from build123d import *

# Parameters (mm, degrees)
F0_W     = 82.55
F0_H     = 190.5
F1_DEPTH = 19.05
F2_W     = 82.55
F2_H     = 25.4
F3_DEPTH = 73.025
F4_R     = 41.27499
F5_R     = 17.4625
F6_DEPTH = 25.4
F8_DEPTH = 25.4


# Not quite as in the source:
# - a fillet or chamfer is up to 0.001 mm smaller than in the source, because OpenCascade refuses the exact size


with BuildPart() as f1:
    # F0 (on Top) → F1 (new body)
    with BuildSketch(Plane.XY):
        with Locations((41.275, 95.25)):
            Rectangle(F0_W, F0_H)
    extrude(amount=F1_DEPTH)

    # F2 (on face) → F3 (join)
    with BuildSketch(Plane.XY.offset(19.05)):
        with Locations((41.275, 177.8)):
            Rectangle(F2_W, F2_H)
    extrude(amount=F3_DEPTH)

    # F4 (radius 41.275 in the source; OpenCascade refuses exactly that, so slightly less here)
    f4_edges = [f1.edges().sort_by_distance(p)[0] for p in [
        (0, 177.8, 92.075),
        (82.55, 177.8, 92.075),
    ]]
    fillet(f4_edges, radius=F4_R)

    # F5 (on face) → F6 (cut)
    with BuildSketch(Plane.XZ.offset(-165.1)):
        with Locations((41.275, 50.8)):
            Circle(F5_R)
    extrude(amount=-F6_DEPTH, mode=Mode.SUBTRACT)

    # F7 (on face) → F8 (cut)
    with BuildSketch(Plane.XY.offset(19.05)):
        with BuildLine():
            ThreePointArc((58.7375, 114.3), (28.9271478335, 126.6478521665), (41.275, 96.8375))
            ThreePointArc((41.275, 96.8375), (53.6228521665, 101.9521478335), (58.7375, 114.3))
        make_face()
        with BuildLine():
            Line((41.275, 38.1), (41.275, 20.6375))
            ThreePointArc((41.275, 20.6375), (53.6228521665, 25.7521478335), (58.7375, 38.1))
            ThreePointArc((58.7375, 38.1), (53.6228521665, 50.4478521665), (41.275, 55.5625))
            Line((41.275, 55.5625), (41.275, 38.1))
        make_face()
        with BuildLine():
            ThreePointArc((41.275, 55.5625), (23.8125, 38.1), (41.275, 20.6375))
            Line((41.275, 20.6375), (41.275, 38.1))
            Line((41.275, 38.1), (41.275, 55.5625))
        make_face()
    extrude(amount=-F8_DEPTH, mode=Mode.SUBTRACT)


solid = f1.part
The model under review builds one solid part; all positions refer to its coordinate system, in mm. A direction names the side the tool comes from. Round coordinates to 2 decimals unless told otherwise and drop trailing zeros. Loops run counter-clockwise (first coordinate to the right, second up) from the corner with the lowest first, then second, coordinate; pieces in that order, holes last. Notation, with made-up numbers: M -17.75,-33 L 3.25,-33 A24 ccw 3.25,-18 Z; hole C 44.5,-40 d11. An arc over 180 degrees is marked long. Answer as CSV lines item,"result".
1. Draft analysis for pull direction X (two halves, no side actions). For faces 3 (the face through (11.77, 177.978, 79.663)), 4 (the face through (32, 190.5, 35)), 5 (the face through (57.4, 177.6, 44.1)), state which applies: pulls with the +X half, pulls with the -X half, needs draft (parallel to the pull), parting line crosses it, or undercut.
Outcome:
face 3,"pulls with the -X half"
face 4,"needs draft"
face 5,"undercut"
2. Insertion check: pin 1 Ø10 at (x, y) = (12.5, 146) entering from +Z; pin 2 Ø22 at (x, z) = (37, 68.5) entering from -Y. Each pin has a flat end and moves straight along its axis. Give the tip position at first contact, or say it passes through.
Outcome:
pin 1,"stops at z = 19.05"
pin 2,"stops at y = 165.1"
3. We need section A-A (z = 48.5). Give the boundary of the cut face in (x, y).
Outcome:
outline,"M 0,165.1 L 23.96,165.1 L 23.96,190.5 L 0,190.5 Z; M 58.59,165.1 L 82.55,165.1 L 82.55,190.5 L 58.59,190.5 Z"
4. We need section D-D (z = 6). Count the separate pieces of the cut face and the enclosed holes in it, plus the area to 3 significant figures.
Outcome:
separate pieces,"1"
enclosed holes,"2"
area,"13,800 mm2"
5. We need section B-B (y = 40). Give the boundary of the cut face in (x, z).
Outcome:
outline,"M 0,0 L 23.92,0 L 23.92,19.05 L 0,19.05 Z; M 58.63,0 L 82.55,0 L 82.55,19.05 L 58.63,19.05 Z"
6. We need section C-C (x = 38.5). Give the boundary of the cut face in (y, z).
Outcome:
outline,"M 0,0 L 20.86,0 L 20.86,19.05 L 0,19.05 Z; M 55.34,0 L 97.06,0 L 97.06,19.05 L 55.34,19.05 Z; M 131.54,0 L 190.5,0 L 190.5,33.56 L 165.1,33.56 L 165.1,19.05 L 131.54,19.05 Z; M 165.1,68.04 L 190.5,68.04 L 190.5,91.98 L 165.1,91.98 Z"
7. For faces 1 (the face through (0, 115, 14)), 2 (the face through (41, 84, 19.05)), list the 3-axis set-ups (+Z, -Z, +X, -X, +Y, -Y) from which the entire face can be reached by the end or side of a thin tool; tool diameter is ignored.
Outcome:
face 1,"+Z, -Z, -X, +Y, -Y"
face 2,"+Z, +X, -X, -Y"
8. To check wall thickness, follow L1, parallel to X at y = 180, z = 50; L2, parallel to Z at x = 51.5, y = 18; L3, parallel to Y at x = 69, z = 36.5. State the ranges of each line that lie inside material, in increasing order. Write a range as [from, to].
Outcome:
L1,"x = [0, 23.83], [58.72, 82.55]"
L2,"z = [0, 19.05]"
L3,"y = [165.1, 190.5]"
